Geometry check sheet. Reference: the model listing, model coordinates, mm. A direction names the side the tool comes from. Round coordinates to 2 decimals unless told otherwise and drop trailing zeros. Order: outer loops, then holes, each group sorted by start corner. A loop starts at its lowest first (then second) coordinate and runs counter-clockwise, first axis right, second up. Notation, with made-up numbers: (-38, 75.25) -> (15, 75.25) arc R22 cw to (15, 104.25) -> close; hole circle Ø5 at (78, -18). An arc over 180 degrees is marked (long way). Answer as a JSON object with one key per item and string values. Group by question number.
Autodesk Fusion 360 part; units mm, degrees
sketch "Sketch1" plane through (0, 0, 0) normal (0, 0, 1) x (1, 0, 0)
  line L0 (22.5, 12.5) -> (-22.5, 12.5)
  line L1 (-22.5, 12.5) -> (-22.5, -12.5)
  line L2 (-22.5, -12.5) -> (22.5, -12.5)
  line L3 (22.5, -12.5) -> (22.5, 12.5)
  line L4 (22.5, 12.5) -> (-22.5, -12.5) construction
  line L5 (-22.5, 12.5) -> (22.5, -12.5) construction
  line L6 (-17.5, 12.5) -> (-17.5, -12.5) construction
  line L7 (0, -12.5) -> (0, 12.5) construction
  line L8 (-22.5, 0) -> (22.5, 0) construction
  line L9 (-20, 7.5) -> (-20, -7.5)
  line L10 (-15, -7.5) -> (-15, 7.5)
  arc A0 (-15, 7.5) -> (-20, 7.5) centre (-17.5, 7.5) ccw
  arc A1 (-20, -7.5) -> (-17.5, -5) centre (-17.5, -7.5) ccw
  line L11 (12.5, 12.5) -> (-12.5, 12.5)
  line L12 (-12.5, 12.5) -> (-12.5, -12.5)
  line L13 (-12.5, -12.5) -> (12.5, -12.5)
  line L14 (12.5, -12.5) -> (12.5, 12.5)
  line L15 (12.5, 12.5) -> (-12.5, -12.5) construction
  line L16 (-12.5, 12.5) -> (12.5, -12.5) construction
  arc A2 (20, 7.5) -> (15, 7.5) centre (17.5, 7.5) ccw
  line L17 (15, -7.5) -> (15, 7.5)
  line L18 (20, 7.5) -> (20, -7.5)
  arc A3 (17.5, -5) -> (20, -7.5) centre (17.5, -7.5) ccw
  dimension "d1" = 45
  dimension "d2" = 25
  dimension "d3" = 5
  dimension "d4" = 5
  dimension "d5" = 5
  dimension "d6" = 15
  dimension "d7" = 25
  dimension "d8" = 25
extrude "Extrude1" add sketch "Sketch1" along normal blind 5 contours L0 L2 L3 L14 | L0 L1 L2 L12 makes body 1 at (13.3333, -2.5, 0) makes body 2 at (-13.3333, -2.5, 0)
extrude "Extrude2" add sketch "Sketch1" along normal blind 15 contours L0 L2 L11 L12 L13 L14 bodies 1 2
sketch "Sketch2" plane through (12.5, 0, 0) normal (1, 0, 0) x (0, 1, 0)
  line L0 (-12.5, 5) -> (12.5, 5)
  line L1 (12.5, 5) -> (12.5, 15)
  line L2 (12.5, 15) -> (-12.5, 15)
  line L3 (-12.5, 15) -> (-12.5, 5)
  line L4 (-12.5, 15) -> (12.5, 15)
  circle A0 centre (0, 28) radius 13
  circle A1 centre (0, 28) radius 18.0347
  line L5 (0, 28) -> (0, 59) construction
  line L6 (-2.5, 40.7574) -> (-2.5, 54.4012)
  line L7 (2.5, 40.7574) -> (2.5, 54.4012)
  line L8 (-7.5, 38.6184) -> (-7.5, 54.4012)
  line L9 (7.5, 38.6184) -> (7.5, 54.4012)
  line L10 (-7.5, 54.4012) -> (-2.5, 54.4012)
  line L11 (2.5, 54.4012) -> (7.5, 54.4012)
  point P0 (0, 15)
  point P1 (7.5, 44.4012)
  dimension "d13" = 26
  dimension "d14" = 36.0694
  dimension "d15" = 5
  dimension "d17" = 5
  dimension "d18" = 5
  dimension "d20" = 10
extrude "Extrude3" add sketch "Sketch2" against normal blind 25 contours L2 L4 A0 A1 L8 | L2 L4 A0 A1 L9 | A1 L6 L8 L10 | A0 A1 L6 L8 | A0 A1 L7 L9 | A1 L7 L9 L11 bodies 1
sketch "Sketch3" plane through (0, -7.5, 0) normal (0, -1, 0) x (1, 0, 0)
  line L0 (12.5, 44.4012) -> (12.5, 54.4012)
  line L1 (12.5, 54.4012) -> (-12.5, 54.4012)
  line L2 (-12.5, 54.4012) -> (-12.5, 44.4012)
  line L3 (-12.5, 44.4012) -> (12.5, 44.4012)
  line L4 (0, 54.4012) -> (0, 44.4012) construction
  line L5 (-12.5, 49.4012) -> (12.5, 49.4012) construction
  circle A0 centre (-7.5, 49.4012) radius 2.5
  circle A1 centre (7.5, 49.4012) radius 2.5
  dimension "d23" = 5
  dimension "d24" = 5
  dimension "d25" = 15
extrude "Extrude4" cut sketch "Sketch3" against normal through all contours A0 | A1 bodies 1
fillet "Fillet1" radius 5 4 edges at (-22.5, 12.5, 2.5) (-22.5, -12.5, 2.5) (22.5, 12.5, 2.5) (22.5, -12.5, 2.5) on bodies 1
fillet "Fillet2" radius 5 4 edges at (12.5, -5, 54.4012) (12.5, 5, 54.4012) (-12.5, -5, 54.4012) (-12.5, 5, 54.4012) on bodies 1
chamfer "Chamfer1" distance 0.5 angle 45 1 faces at (-5, -2.5, 0) on bodies 1
Item 1: Sectioned sample at D-D, the plane x = -11. Enter the section's corners in (y, z).
Item 2: Set-up check for faces 5 (the flat face through (0, 2.5, 47)), 6 (the flat face through (-14, 0, 5)), 7 (the flat face through (0, 12.5, 8)): record each of +Z, -Z, +X, -X, +Y, -Y from which the full face is reachable in a straight line by a thin tool's end or side.
Item 3: Thickness scan on L1, parallel to Y at x = 10, z = 46; L2, parallel to Z at x = 7.5, y = -5; L3, parallel to Y at x = -3, z = 28. Record the ranges inside material, lowest first.
Item 4: Depth check by flat-ended pin: pin 1 Ø11 at (x, z) = (-3.5, 48) entering from +Y; pin 2 Ø4 at (x, z) = (-7.5, 49.4) entering from -Y (3 decimals); pin 3 Ø7 at (x, z) = (-1.5, 5.5) entering from +Y; pin 4 Ø4 at (x, z) = (6.5, 40) entering from +Y. Enter the tip coordinate at first touch or a pass-through.
Item 5: Sectioned sample at B-B, the plane y = 5.5. Count the separate pieces of the cut face and the enclosed holes in it, then the cut area to 3 significant figures.
Item 6: Sectioned sample at C-C, the plane z = 3.5. Enter the section's corners in (x, y), then the cut area to 3 significant figures.
Item 7: Mould release check, pull along X, two halves, no side actions. Record for faces 1 (the cylindrical face through (21.07, 11, 2.78)), 2 (the flat face through (-15, 0, 3)), 3 (the cylindrical face through (6.96, 4.96, 46.96)), 4 (the flat face through (0, 0, 0)): pulls with the +X half, pulls with the -X half, needs draft (parallel to the pull), parting line crosses it, or undercut.
Item 8: Sectioned sample at A-A, the plane z = 28. Enter the section's corners in (x, y).
Result:
{
 "1": {"outline": "(-12.5, 0.5) -> (-12, 0) -> (12, 0) -> (12.5, 0.5) -> (12.5, 15) arc R18.03 ccw to (7.5, 44.4) -> (7.5, 52.97) -> (2.5, 52.97) -> (2.5, 40.76) arc R13 cw (long way) to (-2.5, 40.76) -> (-2.5, 52.97) -> (-7.5, 52.97) -> (-7.5, 44.4) arc R18.03 ccw to (-12.5, 15) -> close"},
 "2": {"face 5": "+Z, +X, -X", "face 6": "+Z, -X, +Y, -Y", "face 7": "-Z, +X, -X, +Y"},
 "3": {"L1": "y = -7.5 to -2.5, 2.5 to 7.5", "L2": "z = 0 to 16, 40 to 46.9, 51.9 to 54.4", "L3": "y = -18.03 to -13, 13 to 18.03"},
 "4": {"pin 1": "stops at y = 10.72", "pin 2": "passes through", "pin 3": "stops at y = 12.5", "pin 4": "stops at y = 15.01"},
 "5": {"separate pieces": "4", "enclosed holes": "2", "area": "770 mm2"},
 "6": {"outline": "(-22.5, -7.5) arc R5 ccw to (-17.5, -12.5) -> (17.5, -12.5) arc R5 ccw to (22.5, -7.5) -> (22.5, 7.5) arc R5 ccw to (17.5, 12.5) -> (-17.5, 12.5) arc R5 ccw to (-22.5, 7.5) -> close; hole (-20, -7.5) arc R2.5 ccw to (-15, -7.5) -> (-15, 7.5) arc R2.5 ccw to (-20, 7.5) -> close; hole (15, -7.5) arc R2.5 ccw to (20, -7.5) -> (20, 7.5) arc R2.5 ccw to (15, 7.5) -> close", "area": "914 mm2"},
 "7": {"face 1": "pulls with the +X half", "face 2": "undercut", "face 3": "undercut", "face 4": "needs draft"},
 "8": {"outline": "(-12.5, -18.03) -> (12.5, -18.03) -> (12.5, -13) -> (-12.5, -13) -> close; (-12.5, 13) -> (12.5, 13) -> (12.5, 18.03) -> (-12.5, 18.03) -> close"}
}
